Work out the finished part from the listing and answer in its coordinate system (mm). A direction names the side the tool comes from. Give positions to 0.01 mm unless a question says otherwise; leave off trailing zeros. Write each loop counter-clockwise with the first axis right and the second up, starting at its lowest first coordinate (ties: lowest second). Pieces come first, ordered by that corner, then holes. Notation, with made-up numbers: (82.5, -19.75) -> (139.5, -19.75) arc R26 ccw to (139.5, 4.25) -> close; hole circle Ø7 at (66, 38). An arc over 180 degrees is marked (long way). Use a Markdown table: item, result. Add a question column.
Q1. For faces 4 (the face through (2, 23, 5)), 5 (the face through (-2.3, 22.6, 0.5)), 6 (the face through (0, 30, 4)), determine the directions among +Z, -Z, +X, -X, +Y, -Y from which every point of the face is accessible in a straight line to the end or side of a thin tool.
Q2. Consider line 1 (Y direction, x = 0.25, z = -3); line 2 (X direction, y = 10, z = 0.5); line 3 (X direction, y = 21, z = 2.25). Determine where each line is inside the solid, lowest interval first.
Q3. Section B-B, the plane z = 5.25 is taken. Give the vertices of the cut face in (x, y), plus the area to 3 significant figures.
Q4. Section C-C, the plane y = 25 is taken. Give the vertices of the cut face in (x, z).
Q5. Section D-D, the plane z = 0 is taken. Give the vertices of the cut face in (x, y).
Q6. For a pull along X with two mould halves and no side action, classify faces 1 (the face through (4.5, 11.46, 8.65)), 2 (the face through (-0.044, 20.744, 5.062)), 3 (the face through (0, 0, 0)) as pulls with the +X half, pulls with the -X half, needs draft (parallel to the pull), parting line crosses it, or undercut.
Q7. Each of these flat-tipped pins is pushed along its axis until it touches: pin 1 Ø1.1 at (y, z) = (23.5, 5.5) entering from +X; pin 2 Ø1.5 at (x, y) = (5.5, 23) entering from -Z; pin 3 Ø8 at (y, z) = (20.5, -1.5) entering from +X. Where does it stop, or does it pass through?
Q8. Section A-A, the plane x = 0 is taken. Give the vertices of the cut face in (y, z).
from build123d import *

# Parameters (mm, degrees)
SKETCH1_R               = 9.75
BOSS_EXTRUDE1_DEPTH     = 30
SKETCH3_W               = 19.5
SKETCH3_H               = 15
CUT_EXTRUDE1_DEPTH      = 0.5
CUT_EXTRUDE1_DEPTH_BACK = 30
CUT_EXTRUDE2_DEPTH      = 30


with BuildPart() as part:
    # Sketch1 → Boss-Extrude1 (new body)
    with BuildSketch(Plane(origin=(0, 0, 0), x_dir=(1, 0, 0), z_dir=(0, 1, 0))):
        Circle(SKETCH1_R)
    extrude(amount=BOSS_EXTRUDE1_DEPTH)

    # Sketch3 → Cut-Extrude1 (cut, two sides)
    with BuildSketch(Plane.XY) as cut_extrude1_sk:
        with Locations((0, 22.5)):
            Rectangle(SKETCH3_W, SKETCH3_H)
    extrude(amount=CUT_EXTRUDE1_DEPTH, mode=Mode.SUBTRACT)
    extrude(cut_extrude1_sk.sketch, amount=-CUT_EXTRUDE1_DEPTH_BACK, mode=Mode.SUBTRACT)

    # Sketch4 → Cut-Extrude2 (cut)
    with BuildSketch(Plane(origin=(0, 0, 0.5), x_dir=(-1, 0, 0), z_dir=(0, 0, -1))):
        with BuildLine():
            Line((2, 23.743843632), (2, 22.743843632))
            ThreePointArc((2, 22.743843632), (0, 20.743843632), (-2, 22.743843632))
            Line((-2, 22.743843632), (-2, 23.743843632))
            ThreePointArc((-2, 23.743843632), (0, 25.743843632), (2, 23.743843632))
        make_face()
    extrude(amount=-CUT_EXTRUDE2_DEPTH, mode=Mode.SUBTRACT)


solid = part.part
Result set:
| question | item | result |
|---|---|---|
| 1 | face 4 | +Z, -Z |
| 1 | face 5 | -Z, +X, -X, +Y |
| 1 | face 6 | +Z, -Z, +X, -X, +Y |
| 2 | line 1 | y = 0 to 15 |
| 2 | line 2 | x = -9.74 to 9.74 |
| 2 | line 3 | x = -9.49 to -0.98, 0.98 to 9.49 |
| 3 | outline | (-8.22, 0) -> (8.22, 0) -> (8.22, 30) -> (-8.22, 30) -> close; hole (-2, 22.74) arc R2 ccw to (2, 22.74) -> (2, 23.74) arc R2 ccw to (-2, 23.74) -> close |
| 3 | area | 476 mm2 |
| 4 | outline | (-9.74, 0.5) -> (-1.56, 0.5) -> (-1.56, 9.62) arc R9.75 ccw to start; (1.56, 0.5) -> (9.74, 0.5) arc R9.75 ccw to (1.56, 9.62) -> close |
| 5 | outline | (-9.75, 0) -> (9.75, 0) -> (9.75, 15) -> (-9.75, 15) -> close |
| 6 | face 1 | parting line crosses it |
| 6 | face 2 | undercut |
| 6 | face 3 | needs draft |
| 7 | pin 1 | stops at x = 8.4 |
| 7 | pin 2 | stops at z = 0.5 |
| 7 | pin 3 | stops at x = 9.74 |
| 8 | outline | (0, -9.75) -> (15, -9.75) -> (15, 0.5) -> (20.74, 0.5) -> (20.74, 9.75) -> (0, 9.75) -> close; (25.74, 0.5) -> (30, 0.5) -> (30, 9.75) -> (25.74, 9.75) -> close |
